Model file for the job. Use its own axes, mm. Give positions to 0.01 mm unless a question says otherwise; leave off trailing zeros. Write each loop counter-clockwise with the first axis right and the second up, starting at its lowest first coordinate (ties: lowest second). Pieces come first, ordered by that corner, then holes. Notation, with made-up numbers: M 79.5,-29.75 L 128.5,-29.75 A27 ccw 128.5,-0.75 Z; hole C 22,-32 d4. An arc over 180 degrees is marked long. Answer as a JSON object with one key per item and string values. Group by question number.
```python
from build123d import *

# Parameters (mm, degrees)
SKETCH_1_R      = 3.4
EXTRUDE_1_DEPTH = 200


with BuildPart() as part:
    # 草图1 → 凸台-拉伸1 (new body)
    with BuildSketch(Plane.XY):
        Polygon((-4.1, 12.5), (-4.1, 15), (-8.25, 15), (-15, 15), (-15, 8.25), (-15, 4.1), (-12.5, 4.1), (-12.5, 8.25), (-9.664213562, 8.25), (-5.8, 4.385786438), (-5.8, -4.385786438), (-9.664213562, -8.25), (-12.5, -8.25), (-12.5, -4.1), (-15, -4.1), (-15, -8.25), (-15, -15), (-8.25, -15), (-4.1, -15), (-4.1, -12.5), (-8.25, -12.5), (-8.25, -9.664213562), (-4.385786438, -5.8), (4.385786438, -5.8), (8.25, -9.664213562), (8.25, -12.5), (4.1, -12.5), (4.1, -15), (8.25, -15), (15, -15), (15, -8.25), (15, -4.1), (12.5, -4.1), (12.5, -8.25), (9.664213562, -8.25), (5.8, -4.385786438), (5.8, 4.385786438), (9.664213562, 8.25), (12.5, 8.25), (12.5, 4.1), (15, 4.1), (15, 8.25), (15, 15), (8.25, 15), (4.1, 15), (4.1, 12.5), (8.25, 12.5), (8.25, 9.664213562), (4.385786438, 5.8), (-4.385786438, 5.8), (-8.25, 9.664213562), (-8.25, 12.5), align=None)
        Circle(SKETCH_1_R, mode=Mode.SUBTRACT)
    extrude(amount=EXTRUDE_1_DEPTH)


solid = part.part
```
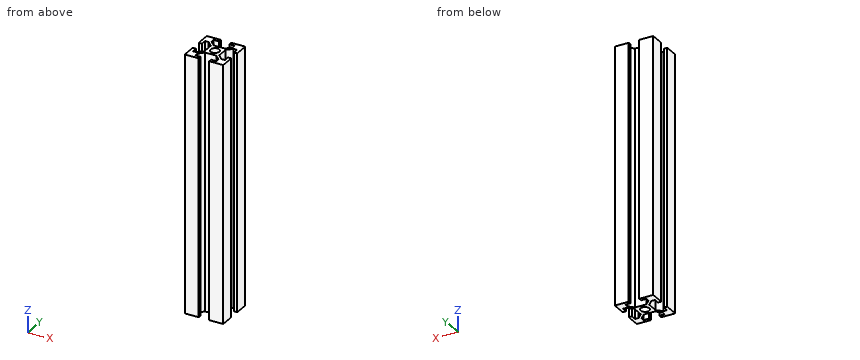
Q1. Wall check: L1, parallel to Y at x = -0.5, z = 22; L2, parallel to Y at x = -11, z = 73; L3, parallel to Y at x = 7, z = 129.5. Give the ranges that are in metal, low to high.
Q2. Drop a flat-ended pin along its axis: P1, Ø4.5, axis at y = -0.5, z = 75.5, coming from the -X side. Give the stop position or say it passes through.
Q3. Slice it at A-A, the plane y = 0. Write the cut outline in (x, z).
Solved:
{
 "1": {"L1": "y = -5.8 to -3.36, 3.36 to 5.8", "L2": "y = -15 to -8.25, 8.25 to 15", "L3": "y = -15 to -12.5, -8.41 to -5.59, 5.59 to 8.41, 12.5 to 15"},
 "2": {"P1": "stops at x = -5.8"},
 "3": {"outline": "M -5.8,0 L -3.4,0 L -3.4,200 L -5.8,200 Z; M 3.4,0 L 5.8,0 L 5.8,200 L 3.4,200 Z"}
}
